```python
from build123d import *

# Parameters (mm, degrees)
SKETCH2_W           = 20
SKETCH2_H           = 20
BOSS_EXTRUDE1_DEPTH = 740
SKETCH3_W           = 19
SKETCH3_H           = 19
CUT_EXTRUDE1_DEPTH  = 740
SKETCH5_R           = 4
CUT_EXTRUDE2_DEPTH  = 20


with BuildPart() as part:
    # Sketch2 → Boss-Extrude1 (new body)
    with BuildSketch(Plane.XY):
        Rectangle(SKETCH2_W, SKETCH2_H)
    extrude(amount=BOSS_EXTRUDE1_DEPTH)

    # Sketch3 → Cut-Extrude1 (cut)
    with BuildSketch(Plane(origin=(0, 0, 0), x_dir=(-1, 0, 0), z_dir=(0, 0, -1))):
        Rectangle(SKETCH3_W, SKETCH3_H)
    extrude(amount=-CUT_EXTRUDE1_DEPTH, mode=Mode.SUBTRACT)

    # Sketch5 → Cut-Extrude2 (cut)
    with BuildSketch(Plane.XZ.offset(10)):
        with Locations(Location((0, 240, 0), (0, 0, 270))):
            Circle(SKETCH5_R)
    extrude(amount=-CUT_EXTRUDE2_DEPTH, mode=Mode.SUBTRACT)


solid = part.part
```
Read the model definition and answer for the solid it produces. Units are mm, in the model's axes. A direction names the side the tool comes from. Coordinates: 2 decimals unless noted, no trailing zeros. Write each loop counter-clockwise with the first axis right and the second up, starting at its lowest first coordinate (ties: lowest second). Pieces come first, ordered by that corner, then holes. Notation, with made-up numbers: (-28, -17.75) -> (-11, -17.75) arc R24 ccw to (-11, 11.25) -> close; hole circle Ø10 at (16, 80.5). An arc over 180 degrees is marked (long way). Answer as a JSON object with one key per item and string values.
Q1. Determine the mould class of faces 1 (the flat face through (0, 9.5, 365)), 2 (the flat face through (-9.5, 0, 365)), 3 (the flat face through (0, 10, 365)), 4 (the flat face through (-10, 0, 365)) for opening direction X: pulls with the +X half, pulls with the -X half, needs draft (parallel to the pull), parting line crosses it, or undercut.
The answers:
{"face 1": "undercut", "face 2": "undercut", "face 3": "needs draft", "face 4": "pulls with the -X half"}
Q2. Consider line 1 (X direction, y = -4.5, z = 693); line 2 (X direction, y = -9.6, z = 240). Determine where each line is inside the solid, lowest interval first. Write a range as [from, to].
The answers:
{"line 1": "x = [-10, -9.5], [9.5, 10]", "line 2": "x = [-10, -4], [4, 10]"}
Q3. The part is cut by section A-A on y = 5.5. Give the vertices of the cut face in (x, z).
The answers:
{"outline": "(-10, 0) -> (-9.5, 0) -> (-9.5, 740) -> (-10, 740) -> close; (9.5, 0) -> (10, 0) -> (10, 740) -> (9.5, 740) -> close"}
Q4. A tool of negligible diameter and unlimited length cuts with its end or side. For faces 5 (the flat face through (0, -10, 365)), 6 (the flat face through (0, -9.5, 365)), from which of +Z, -Z, +X, -X, +Y, -Y can it reach the whole face along a straight path? Write none if from no direction.
The answers:
{"face 5": "+Z, -Z, +X, -X, -Y", "face 6": "+Z, -Z"}
Q5. The part is cut by section B-B on z = 369. Give the vertices of the cut face in (x, y).
The answers:
{"outline": "(-10, -10) -> (10, -10) -> (10, 10) -> (-10, 10) -> close; hole (-9.5, -9.5) -> (9.5, -9.5) -> (9.5, 9.5) -> (-9.5, 9.5) -> close"}
